The model under review builds one solid part; all positions refer to its coordinate system, in mm. Give positions to 0.01 mm unless a question says otherwise; leave off trailing zeros. Order: outer loops, then holes, each group sorted by start corner. A loop starts at its lowest first (then second) coordinate and runs counter-clockwise, first axis right, second up.
Autodesk Inventor part; units mm, degrees
ref_plane "YZ Plane" through (0, 0, 0) normal (1, 0, 0) x (0, 1, 0)
ref_plane "XZ Plane" through (0, 0, 0) normal (0, 1, 0) x (-1, 0, 0)
ref_plane "XY Plane" through (0, 0, 0) normal (0, 0, 1) x (1, 0, 0)
sketch "Sketch1" plane through (0, 0, 0) normal (0, 1, 0) x (-1, 0, 0)
  line L0 (0, 0) -> (750, 0)
  line L1 (750, 0) -> (750, -1500)
  line L2 (750, -1500) -> (0, -1500)
  line L3 (0, -1500) -> (0, 0)
  line L4 (750, -1500) -> (750, -1480)
  line L5 (750, -1480) -> (0, -1480)
  line L6 (0, -1500) -> (750, -1500)
  line L7 (0, 0) -> (0, -20)
  line L8 (0, -20) -> (750, -20)
  line L9 (750, 0) -> (0, 0)
  dimension "d2" = 750
  dimension "d3" = 1500
  dimension "d6" = 20
  dimension "d7" = 20
extrude "Extrusion1" add sketch "Sketch1" along normal blind 50
sketch "Sketch2" plane through (0, 0, 0) normal (0, -1, 0) x (1, 0, 0)
  line L0 (0, 0) -> (0, -1500)
  line L1 (-750, -1500) -> (-750, 0)
  line L2 (0, 0) -> (-750, 0)
  line L3 (-750, 0) -> (-750, -20)
  line L4 (-750, -20) -> (0, -20)
  line L5 (0, -20) -> (0, 0)
  line L6 (0, -1500) -> (-750, -1500)
  line L7 (-750, -1500) -> (-750, -1480)
  line L8 (-750, -1480) -> (0, -1480)
  line L9 (0, -1480) -> (0, -1500)
  dimension "d8" = 20
  dimension "d9" = 20
extrude "Extrusion2" cut sketch "Sketch2" against normal blind 20 contours L0 L4 L1 L2 | L0 L6 L1 L8
sketch "Sketch3" plane through (0, 0, 0) normal (0, -1, 0) x (1, 0, 0)
  line L0 (0, -20) -> (0, -1480)
  circle A0 centre (-562, -20) radius 5
  circle A1 centre (-375, -20) radius 5
  circle A2 centre (-188, -20) radius 5
  line L1 (-750, -1480) -> (0, -1480)
  line L2 (-188, -20) -> (1272, -20) construction
  line L3 (-375, -20) -> (1085, -20) construction
  line L4 (0, -20) -> (-750, -20)
  line L5 (-562, -20) -> (898, -20) construction
  circle A3 centre (-562, -1480) radius 5
  circle A4 centre (-375, -1480) radius 5
  circle A5 centre (-188, -1480) radius 5
  point P0 (0, 0)
  dimension "d15" = 10
  dimension "d16" = 10
  dimension "d17" = 10
  dimension "d24" = 10
  dimension "d25" = 10
  dimension "d26" = 10
extrude "Extrusion3" cut sketch "Sketch3" against normal blind 61.275
thread "Thread1"
thread "Thread2"
thread "Thread3"
thread "Thread4"
thread "Thread5"
thread "Thread6"
sketch "Sketch4" plane through (0, 50, 0) normal (0, 1, 0) x (1, 0, 0)
  line L0 (-650, 1000) -> (-350, 1000)
  line L1 (-350, 1000) -> (-350, 920)
  line L2 (-350, 920) -> (-650, 920)
  line L3 (-650, 920) -> (-650, 1000)
  point P0 (0, 0)
  point P1 (-750, 1500)
  dimension "d47" = 300
  dimension "d48" = 80
extrude "Extrusion4" cut sketch "Sketch4" against normal blind 220.025
properties part number "bench"
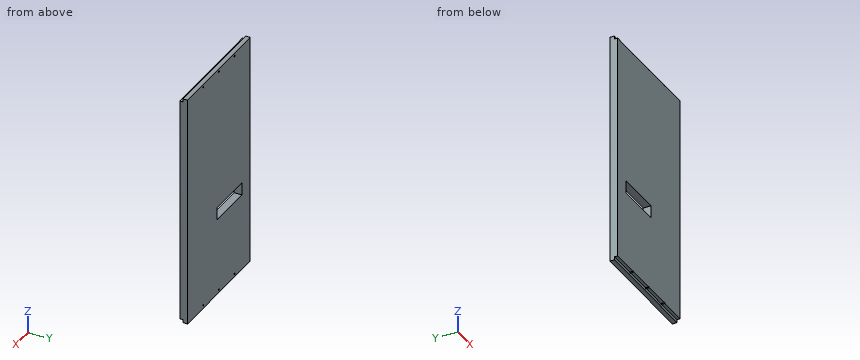
Item 1: Take a section at B-B (y = 36). Give the boundary of the cut face in (x, z).
Values found:
outline: (-750, -1500) - (0, -1500) - (0, 0) - (-750, 0) - close; hole (-650, -1000) - (-350, -1000) - (-350, -920) - (-650, -920) - close; hole circle Ø10 at (-562, -1480); hole circle Ø10 at (-562, -20); hole circle Ø10 at (-375, -1480); hole circle Ø10 at (-375, -20); hole circle Ø10 at (-188, -1480); hole circle Ø10 at (-188, -20)
Item 2: Take a section at A-A (x = -425.5). Give the boundary of the cut face in (y, z), and give its area (3 significant figures).
Values found:
outline: (0, -1480) - (20, -1480) - (20, -1500) - (50, -1500) - (50, -1000) - (0, -1000) - close; (0, -920) - (50, -920) - (50, 0) - (20, 0) - (20, -20) - (0, -20) - close
area: 70,200 mm2
Item 3: Clearance check with flat-ended pins moving along their axes: pin 1 Ø6 at (x, z) = (-562, -20) entering from -Y; pin 2 Ø22 at (x, z) = (-414.5, -5.5) entering from -Y; pin 3 Ø6 at (x, y) = (-116.5, 10) entering from -Z; pin 4 Ø16 at (x, y) = (-647, 11) entering from +Z. State where each tip first meets the part, or that it passes through.
Values found:
pin 1: passes through
pin 2: stops at y = 20
pin 3: stops at z = -1480
pin 4: stops at z = -20
Item 4: For line 1 (X direction, y = 32.5, z = -1480); line 2 (Z direction, x = -479, y = 5); line 3 (X direction, y = 36, z = -957.5), list the stretches that pass through material, from the lowest coordinate up.
Values found:
line 1: x = -750 to -567, -557 to -380, -370 to -193, -183 to 0
line 2: z = -1480 to -1000, -920 to -20
line 3: x = -750 to -650, -350 to 0
